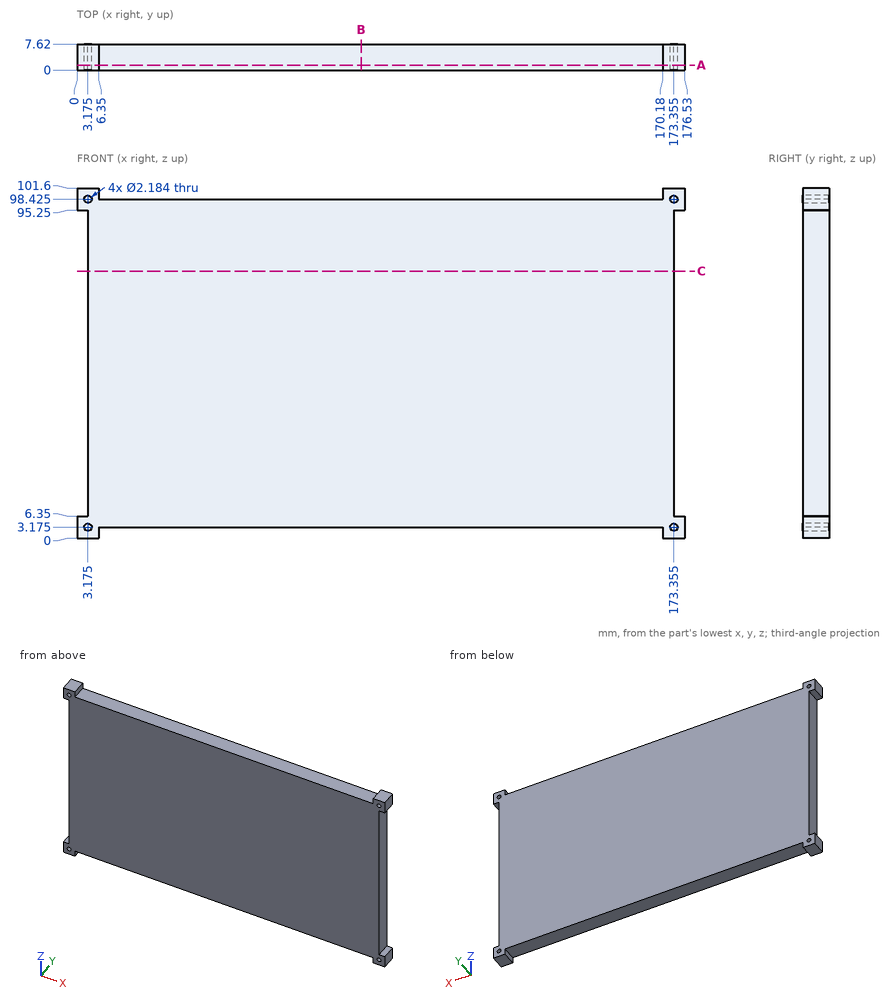
Print and shaded views of the part. All mm, measured from the part's lowest x, y and z. Round coordinates to 2 decimals unless told otherwise and drop trailing zeros. Write each loop counter-clockwise with the first axis right and the second up, starting at its lowest first coordinate (ties: lowest second). Pieces come first, ordered by that corner, then holes. Notation, with made-up numbers: (-39.5, 5.25) - (-9.5, 5.25) arc R16 ccw to (-9.5, 23.25) - close; hole circle Ø8 at (87.25, -14.5). An arc over 180 degrees is marked (long way). Write each question's results on one line, items separated by ' | '. Start each with the question number.
Item 1: Saw through at A-A (y = 1.5). State how many separate pieces and enclosed holes the cut face has, and give its area (3 significant figures).
Item 2: Drop flat-ended pins along their axis: P1, Ø4, axis at y = 5, z = 48.5, coming from the +X side (3 decimals); P2, Ø4, axis at x = 65.5, y = 5, coming from the +Z side (3 decimals); P3, Ø2.5, axis at y = 2.5, z = 49.5, coming from the -X side (3 decimals). Give the stop position or say it passes through.
Item 3: Saw through at B-B (x = 82.5). Write the cut outline in (y, z) (1 decimal), and give its area (3 significant figures).
Item 4: Wall check: L1, parallel to Z at x = 125.5, y = 0.75 (1 decimal); L2, parallel to X at y = 1.75, z = 15.5 (1 decimal). Give the ranges that are in metal, low to high. Write a range as [from, to].
Item 5: Saw through at C-C (z = 77.5). Write the cut outline in (x, y) (1 decimal), and give its area (3 significant figures).
Results are:
1) separate pieces: 1 | enclosed holes: 4 | area: 16,300 mm²
2) P1: stops at x = 173.355 | P2: stops at z = 98.425 | P3: stops at x = 3.175
3) outline: (0, 3.2) - (7.6, 3.2) - (7.6, 98.4) - (0, 98.4) - close | area: 726 mm²
4) L1: z = [3.2, 98.4] | L2: x = [3.2, 173.4]
5) outline: (3.2, 0) - (173.4, 0) - (173.4, 7.6) - (3.2, 7.6) - close | area: 1,300 mm²
